Here's how the part is built. I have some questions about the finished solid (model axes, mm). A direction names the side the tool comes from. Coordinates: 2 decimals unless noted, no trailing zeros. Write each loop counter-clockwise with the first axis right and the second up, starting at its lowest first coordinate (ties: lowest second). Pieces come first, ordered by that corner, then holes.
from build123d import *

# Parameters (mm, degrees)
F0_W     = 63.609058
F0_H     = 44.548504
F1_DEPTH = 19.05
F3_DEPTH = 19.05
F4_W     = 44.548504
F4_H     = 19.05
F5_DEPTH = 19.05


with BuildPart() as f1:
    # F0 (on Top) → F1 (new body)
    with BuildSketch(Plane.XY):
        with Locations((-22.052619, 7.86802)):
            Rectangle(F0_W, F0_H)
    extrude(amount=F1_DEPTH)

    # F2 (on face) → F3 (join)
    with BuildSketch(Plane(origin=(-53.857148, 0, 0), x_dir=(0, -1, 0), z_dir=(-1, 0, 0))):
        Polygon((-49.093768, 0), (14.406232, 0), (14.406232, 44.45), (-4.643768, 44.45), (-49.093768, 12.700002), align=None)
    extrude(amount=F3_DEPTH)

    # F4 (on face) → F5 (join)
    with BuildSketch(Plane.YZ.offset(9.75191)):
        Polygon((-14.406232, 44.45), (-14.406232, 19.05), (30.142272, 19.05), (30.142272, 0), (49.093768, 0), (49.093768, 12.7), (4.643768, 44.45), align=None)
        with Locations((7.86802, 9.525)):
            Rectangle(F4_W, F4_H)
    extrude(amount=F5_DEPTH)


solid = f1.part
1. If I drill on line 1 (X direction, y = 30.5, z = 19); line 2 (Y direction, x = -23, z = 13); line 3 (Z direction, x = -22, y = 2), over which ranges is the centre line in solid material (lowest first)?
2. I want a section at C-C (z = 36.5). List the corners of the cut face in (x, y) for me, then the cut area to 3 significant figures.
3. For pin 1 Ø2 at (x, y) = (-61.5, 35) entering from +Z; pin 2 Ø10 at (x, y) = (18.5, 11) entering from +Z; pin 3 Ø3 at (x, y) = (-37.5, 23.5) entering from +Z, each with a flat end and sliding along its axis, tell me the tip position at first contact or that it passes through.
4. I want a section at D-D (y = -9.5). List the corners of the cut face in (x, z) for me, then the cut area to 3 significant figures.
5. Thinking about a two-plate mould opening in X: for faces 6 (the face through (-53.857, 18, 23)), 7 (the face through (-23, -14.406, 18)), 8 (the face through (28.802, 10, 18)), 9 (the face through (-72.907, 11, 18)), which applies, pulls with the +X half, pulls with the -X half, needs draft (parallel to the pull), parting line crosses it, or undercut?
6. I want a section at B-B (y = 43.5). List the corners of the cut face in (x, z) for me.
7. On a 3-axis mill with a long thin cutter (end or side, diameter ignored), from which of +Z, -Z, +X, -X, +Y, -Y can I reach the whole of each face in a straight line? I mean faces 1 (the face through (-23, 10, 0)), 2 (the face through (-22, 8, 19.05)), 3 (the face through (-63.249, 26.558, 28.797)), 4 (the face through (9.752, 17, 23)), 5 (the face through (-22, 30.142, 9)). Say none if no direction works.
8. I want a section at A-A (z = 10.5). List the corners of the cut face in (x, y) for me, then the cut area to 3 significant figures.
Response values:
1. line 1: x = -72.91 to -53.86, 9.75 to 28.8
1. line 2: y = -14.41 to 30.14
1. line 3: z = 0 to 19.05
2. outline: (-72.91, -14.41) - (-53.86, -14.41) - (-53.86, 15.77) - (-72.91, 15.77) - close; (9.75, -14.41) - (28.8, -14.41) - (28.8, 15.77) - (9.75, 15.77) - close
2. area: 1,150 mm2
3. pin 1: stops at z = 23.48
3. pin 2: stops at z = 43.48
3. pin 3: stops at z = 19.05
4. outline: (-72.91, 0) - (28.8, 0) - (28.8, 44.45) - (9.75, 44.45) - (9.75, 19.05) - (-53.86, 19.05) - (-53.86, 44.45) - (-72.91, 44.45) - close
4. area: 2,910 mm2
5. face 6: undercut
5. face 7: needs draft
5. face 8: pulls with the +X half
5. face 9: pulls with the -X half
6. outline: (-72.91, 0) - (-53.86, 0) - (-53.86, 16.7) - (-72.91, 16.7) - close; (9.75, 0) - (28.8, 0) - (28.8, 16.7) - (9.75, 16.7) - close
7. face 1: -Z, +X, -X, +Y, -Y
7. face 2: +Z, +Y, -Y
7. face 3: +Z, +X, -X, +Y
7. face 4: +Z, +Y
7. face 5: +Z, -Z, +Y
8. outline: (-72.91, -14.41) - (28.8, -14.41) - (28.8, 49.09) - (9.75, 49.09) - (9.75, 30.14) - (-53.86, 30.14) - (-53.86, 49.09) - (-72.91, 49.09) - close
8. area: 5,250 mm2
